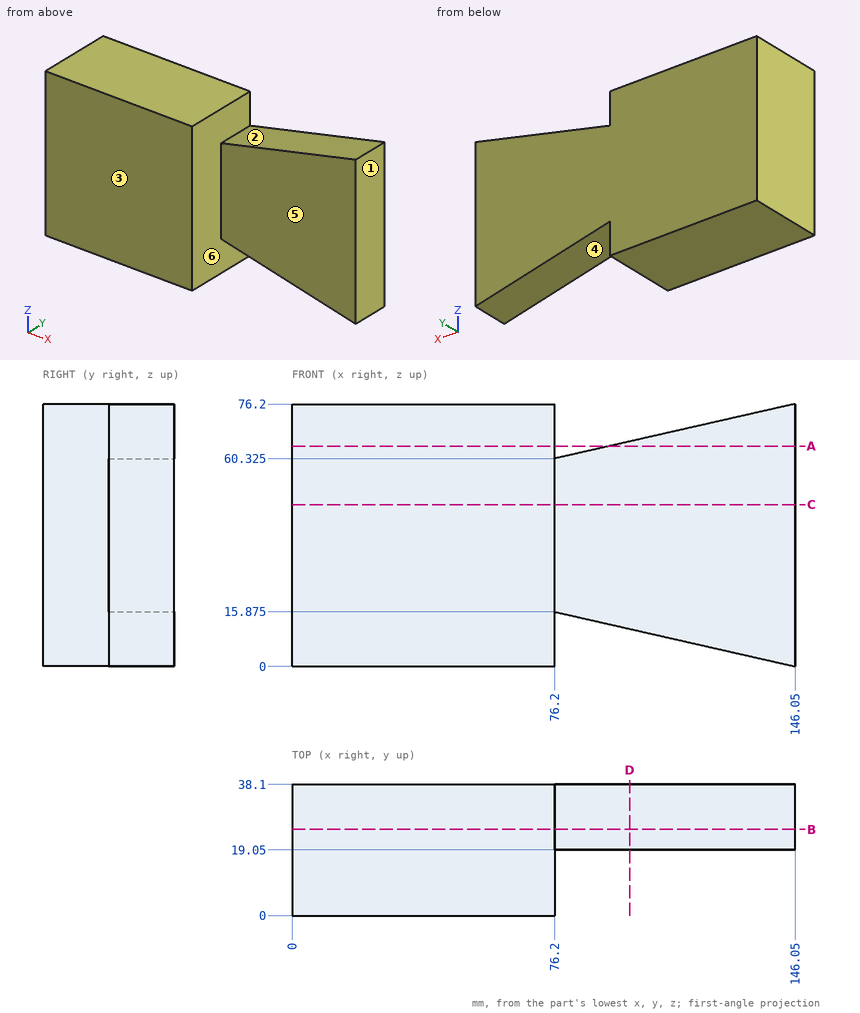
Here's the drawing with two shaded views (mm, measured from the low corner). I have some questions. A direction names the side the tool comes from. Round coordinates to 2 decimals unless told otherwise and drop trailing zeros. Loops run counter-clockwise (first coordinate to the right, second up) from the corner with the lowest first, then second, coordinate; pieces in that order, holes last. Notation, with made-up numbers: (81.25, -31) - (120.25, -31) arc R28 ccw to (120.25, 3) - close; hole circle Ø10 at (77.5, -31). An arc over 180 degrees is marked (long way). Use CSV: the item, a comma, the result in double quotes. Start each with the question number.
1) If we section it at C-C on z = 47: Write out the boundary of the cut face in (x, y), plus the area to 3 significant figures.
2) For pin 1 Ø8 at (x, y) = (81, 29.5) entering from +Z (3 decimals); pin 2 Ø5 at (x, y) = (94, 28) entering from +Z; pin 3 Ø1.5 at (y, z) = (7, 14.5) entering from +X, each with a flat end and sliding along its axis, tell me the tip position at first contact or that it passes through.
3) Please list where these lines run through material, in increasing order: probe 1 along X at (y, z) = (2, 69); probe 2 along Y at (x, z) = (125, 56); probe 3 along Z at (x, y) = (106, 31). Write a range as [from, to].
4) If we section it at D-D on x = 98: Write out the boundary of the cut face in (y, z).
5) For the marked faces 4, 5 and 6, which set-ups out of +Z, -Z, +X, -X, +Y, -Y let a thin tool reach every point of the face, with its end or its side?
6) If we section it at B-B on y = 25: Write out the boundary of the cut face in (x, z) (3 decimals), plus the area to 3 significant figures.
7) If we section it at A-A on z = 64: Write out the boundary of the cut face in (x, y), plus the area to 3 significant figures.
8) We'd pull the mould along X, two halves only. Please class the marked faces 1, 2 and 3: released by +X, released by -X, zero draft, split by the parting line, or undercut.
Geometry results:
1,outline,"(0, 0) - (76.2, 0) - (76.2, 19.05) - (146.05, 19.05) - (146.05, 38.1) - (0, 38.1) - close"
1,area,"4,230 mm2"
2,pin 1,"stops at z = 62.325"
2,pin 2,"stops at z = 64.94"
2,pin 3,"stops at x = 76.2"
3,probe 1,"x = [0, 76.2]"
3,probe 2,"y = [19.05, 38.1]"
3,probe 3,"z = [9.1, 67.1]"
4,outline,"(19.05, 10.92) - (38.1, 10.92) - (38.1, 65.28) - (19.05, 65.28) - close"
5,face 4,"-Z, +Y, -Y"
5,face 5,"+Z, -Z, +X, -Y"
5,face 6,"-Y"
6,outline,"(0, 0) - (76.2, 0) - (76.2, 15.875) - (146.05, 0) - (146.05, 76.2) - (76.2, 60.325) - (76.2, 76.2) - (0, 76.2) - close"
6,area,"10,000 mm2"
7,outline,"(0, 0) - (76.2, 0) - (76.2, 38.1) - (0, 38.1) - close; (92.37, 19.05) - (146.05, 19.05) - (146.05, 38.1) - (92.37, 38.1) - close"
7,area,"3,930 mm2"
8,face 1,"released by +X"
8,face 2,"undercut"
8,face 3,"zero draft"
